Design review of the part built by this model. Coordinates are the model's own, in mm. Coordinates: 2 decimals unless noted, no trailing zeros. Loops run counter-clockwise (first coordinate to the right, second up) from the corner with the lowest first, then second, coordinate; pieces in that order, holes last. Notation, with made-up numbers: (78.5, 36) - (111.5, 36) arc R25 ccw to (111.5, 69) - close; hole circle Ø5 at (57.5, -24.75). An arc over 180 degrees is marked (long way). Use one line per item in the form item = value. Start each with the question number.
(1) Add section A-A (y = 2.25). State the section outline as (x, z) points.
(2) Clearance check with flat-ended pins moving along their axes: pin 1 Ø4 at (x, y) = (14, 9) entering from -Z; pin 2 Ø12 at (x, z) = (-15.24, 218.44) entering from +Y; pin 3 Ø6 at (x, z) = (15.24, 187.96) entering from +Y; pin 4 Ø5 at (x, y) = (-18, 10.5) entering from +Z. State where each tip first meets the part, or that it passes through.
(3) Add section B-B (z = -169.5). State the section outline as (x, y) points (1 decimal), plus the area to 3 significant figures.
(4) For L1, parallel to Z at x = 0, y = 8.25; L2, parallel to X at y = 2.3, z = 218.44; L3, parallel to X at y = 7.05, z = 187.96, list the stretches that pass through material, from the lowest coordinate up.
```python
from build123d import *

# Parameters (mm, degrees)
SKETCH1_W               = 50.8
SKETCH1_H               = 457.2
BOSS_EXTRUDE1_DEPTH     = 12.7
SKETCH2_R               = 4.7625
CUT_EXTRUDE1_DEPTH      = 76.2
F_1_4_CLEARANCE_HOLE1_D = 6.7564
SKETCH11_R              = 13.208
CUT_EXTRUDE2_DEPTH      = 1.5875
SKETCH13_R              = 3.81
CUT_EXTRUDE3_DEPTH      = 231.35713577
SKETCH15_W              = 17.78
SKETCH15_H              = 15.24
SKETCH15_H_2            = 17.78
CUT_EXTRUDE4_DEPTH      = 4.7625
SKETCH16_R              = 6.858
CUT_EXTRUDE5_DEPTH      = 4.7625


with BuildPart() as part:
    # Sketch1 → Boss-Extrude1 (new body)
    with BuildSketch(Plane(origin=(0, 0, 0), x_dir=(1, 0, 0), z_dir=(0, 1, 0))):
        Rectangle(SKETCH1_W, SKETCH1_H)
    extrude(amount=BOSS_EXTRUDE1_DEPTH)

    # Sketch2 → Cut-Extrude1 (cut)
    with BuildSketch(Plane(origin=(0, 0, -228.6), x_dir=(-1, 0, 0), z_dir=(0, 0, -1))):
        with Locations((-12.7, 12.7)):
            Circle(SKETCH2_R)
        with Locations((12.7, 12.7)):
            Circle(SKETCH2_R)
        with Locations((-12.7, 0)):
            Circle(SKETCH2_R)
        with Locations((12.7, 0)):
            Circle(SKETCH2_R)
    extrude(amount=-CUT_EXTRUDE1_DEPTH, mode=Mode.SUBTRACT)

    # 1/4 Clearance Hole1 (through all)
    with Locations(Plane(origin=(0, 12.7, 0), x_dir=(1, 0, 0), z_dir=(0, 1, 0))):
        with Locations((0, 203.2), (0, 177.8), (25.4, 203.2), (25.4, 177.8), (-25.4, 177.8), (-25.4, 203.2)):
            Hole(F_1_4_CLEARANCE_HOLE1_D / 2)

    # Sketch11 → Cut-Extrude2 (cut)
    with BuildSketch(Plane(origin=(0, 12.7, 0), x_dir=(1, 0, 0), z_dir=(0, 1, 0))):
        with Locations(Location((0, -203.2, 0), (0, 0, 270))):
            Circle(SKETCH11_R)
    extrude(amount=-CUT_EXTRUDE2_DEPTH, mode=Mode.SUBTRACT)

    # Sketch13 → Cut-Extrude3 (cut, through all)
    with BuildSketch(Plane(origin=(0, 12.7, 0), x_dir=(1, 0, 0), z_dir=(0, 1, 0))):
        with Locations(Location((-15.24, -187.96, 0), (0, 0, 270))):
            Circle(SKETCH13_R)
        with Locations(Location((15.24, -187.96, 0), (0, 0, 270))):
            Circle(SKETCH13_R)
        with Locations(Location((15.24, -218.44, 0), (0, 0, 270))):
            Circle(SKETCH13_R)
        with Locations(Location((-15.24, -218.44, 0), (0, 0, 270))):
            Circle(SKETCH13_R)
    extrude(amount=-CUT_EXTRUDE3_DEPTH, mode=Mode.SUBTRACT)

    # Sketch15 → Cut-Extrude4 (cut)
    with BuildSketch(Plane(origin=(0, 12.7, 0), x_dir=(1, 0, 0), z_dir=(0, 1, 0))):
        with Locations((-16.51, -187.96)):
            Rectangle(SKETCH15_W, SKETCH15_H)
        with Locations((16.51, -187.96)):
            Rectangle(SKETCH15_W, SKETCH15_H)
        with Locations((-16.51, -219.71)):
            Rectangle(SKETCH15_W, SKETCH15_H_2)
        with Locations((16.51, -219.71)):
            Rectangle(SKETCH15_W, SKETCH15_H_2)
    extrude(amount=-CUT_EXTRUDE4_DEPTH, mode=Mode.SUBTRACT)

    # Sketch16 → Cut-Extrude5 (cut)
    with BuildSketch(Plane.XZ):
        with Locations(Location((-15.24, 218.44, 0), (0, 0, 270))):
            Circle(SKETCH16_R)
        with Locations(Location((15.24, 218.44, 0), (0, 0, 270))):
            Circle(SKETCH16_R)
        with Locations(Location((15.24, 187.96, 0), (0, 0, 270))):
            Circle(SKETCH16_R)
        with Locations(Location((-15.24, 187.96, 0), (0, 0, 270))):
            Circle(SKETCH16_R)
    extrude(amount=-CUT_EXTRUDE5_DEPTH, mode=Mode.SUBTRACT)


solid = part.part
```
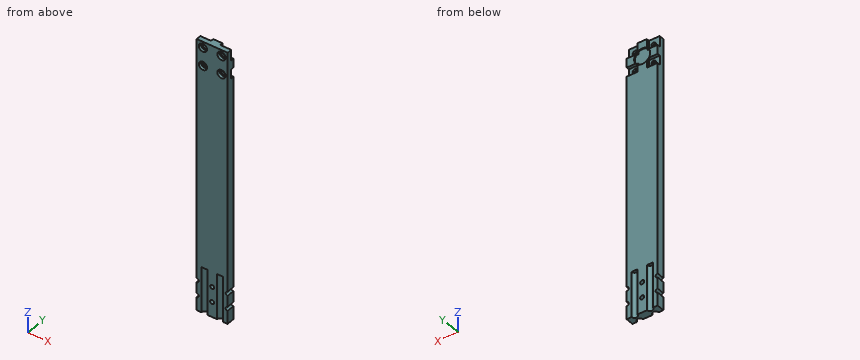
Computed values:
q1.outline = (-25.4, -228.6) - (-16.9, -228.6) - (-16.9, -152.4) - (-8.5, -152.4) - (-8.5, -228.6) - (8.5, -228.6) - (8.5, -152.4) - (16.9, -152.4) - (16.9, -228.6) - (25.4, -228.6) - (25.4, -206.58) arc R3.38 cw to (25.4, -199.82) - (25.4, -181.18) arc R3.38 cw to (25.4, -174.42) - (25.4, 228.6) - (-25.4, 228.6) - (-25.4, -174.42) arc R3.38 cw to (-25.4, -181.18) - (-25.4, -199.82) arc R3.38 cw to (-25.4, -206.58) - close; hole circle Ø13.72 at (-15.24, 187.96); hole circle Ø13.72 at (-15.24, 218.44); hole circle Ø6.76 at (0, -203.2); hole circle Ø6.76 at (0, -177.8); hole circle Ø13.72 at (15.24, 187.96); hole circle Ø13.72 at (15.24, 218.44)
q2.pin_1 = -228.6
q2.pin_2 = 7.94
q2.pin_3 = through
q2.pin_4 = 210.82
q3.outline = (-25.4, 0) - (-17.5, 0) arc R4.8 cw to (-7.9, 0) - (7.9, 0) arc R4.8 cw to (17.5, 0) - (25.4, 0) - (25.4, 12.7) - (17.5, 12.7) arc R4.8 cw to (7.9, 12.7) - (-7.9, 12.7) arc R4.8 cw to (-17.5, 12.7) - (-25.4, 12.7) - close
q3.area = 503 mm^2
q4.L1 = -228.6 to -206.58, -199.82 to -181.18, -174.42 to 228.6
q4.L2 = -25.4 to -22.1, -8.38 to 8.38, 22.1 to 25.4
q4.L3 = -25.4 to -19.05, -11.43 to 11.43, 19.05 to 25.4
